```python
from build123d import *

# Parameters (mm, degrees)
SKETCH2_R           = 1.5
BOSS_EXTRUDE1_DEPTH = 23.04
FILLET1_R           = 0.1


with BuildPart() as part:
    # Sketch1 → Revolve1 (revolve)
    with BuildSketch(Plane(origin=(0, 0, 0), x_dir=(0, 0, -1), z_dir=(1, 0, 0))):
        Polygon((618.283966683, 10.92855784), (618.283966683, 7.778306403), (647.128456403, 7.778306403), (647.128456403, 60.052791184), (640.335726742, 60.052791184), (640.335726742, 55.130523314), (637.579256734, 55.130523314), align=None)
    revolve(axis=Axis((0, 60.052791184, -647.128456403), (0, -1, 0)))

    # Sketch2 → Boss-Extrude1 (add)
    with BuildSketch(Plane(origin=(0, 60.052791184, 0), x_dir=(1, 0, 0), z_dir=(0, 1, 0))):
        with Locations(Location((0, 651.328456403, 0), (0, 0, 90))):
            Circle(SKETCH2_R)
        with Locations(Location((-4.2, 647.128456403, 0), (0, 0, 90))):
            Circle(SKETCH2_R)
        with Locations(Location((0, 642.928456403, 0), (0, 0, 90))):
            Circle(SKETCH2_R)
        with Locations(Location((4.2, 647.128456403, 0), (0, 0, 90))):
            Circle(SKETCH2_R)
    extrude(amount=BOSS_EXTRUDE1_DEPTH)

    # Fillet1
    fillet1_edges = [part.edges().sort_by_distance(p)[0] for p in [
        (0, 60.052791184, -641.428456403),
    ]]
    fillet(fillet1_edges, radius=FILLET1_R)


solid = part.part
```
Work out the finished part from the listing and answer in its coordinate system (mm). A direction names the side the tool comes from. Round coordinates to 2 decimals unless told otherwise and drop trailing zeros. Write each loop counter-clockwise with the first axis right and the second up, starting at its lowest first coordinate (ties: lowest second). Pieces come first, ordered by that corner, then holes.
1) Which of the six approach directions +Z, -Z, +X, -X, +Y, -Y give full straight-line access (tool end or side, diameter ignored) to faces 4 (the face through (-4.65, 71.41, -648.56)), 5 (the face through (0, 7.778, -648))?
2) Consider probe 1 along Y at (x, z) = (-22, -639); probe 2 along Y at (x, z) = (-20.5, -656); probe 3 along X at (y, z) = (23, -629). Determine where each line is inside the solid, lowest interval first.
3) Flat-ended cylindrical pins translate along their axes: P1, Ø8, axis at x = -8, z = -642, coming from the +Y side; P2, Ø10, axis at x = -8, y = 22.5, coming from the +Z side; P3, Ø3, axis at x = -7.5, y = 37, coming from the +Z side. Find the tip coordinate at first contact, or state that the pin passes through.
4) A cutting plane is placed at C-C on y = 48.5. Determine the outline of the cut face in (x, z), and give its area (3 significant figures).
5) A cutting plane is placed at A-A on x = 0. Determine the outline of the cut face in (y, z).
6) Determine the mould class of faces 1 (the face through (0, 83.093, -651)), 2 (the face through (-0.07, 71.46, -641.43)), 3 (the face through (0, 60.053, -647)) for opening direction X: pulls with the +X half, pulls with the -X half, needs draft (parallel to the pull), parting line crosses it, or undercut.
7) A cutting plane is placed at B-B on y = 65.5. Determine the outline of the cut face in (x, z), and give its area (3 significant figures).
Entries:
1. face 4: +Y
1. face 5: +Z, -Z, +X, -X, -Y
2. probe 1: y = 7.78 to 23.28
2. probe 2: y = 7.78 to 25.84
2. probe 3: x = -15.07 to 15.07
3. P1: stops at y = 60.05
3. P2: stops at z = -622.04
3. P3: stops at z = -630.39
4. outline: circle Ø24.89 at (0, -647.13)
4. area: 486 mm2
5. outline: (7.78, -675.97) - (10.93, -675.97) - (55.13, -656.68) - (55.13, -653.92) - (60.05, -653.92) - (60.05, -652.83) - (83.09, -652.83) - (83.09, -649.83) - (60.05, -649.83) - (60.05, -644.53) arc R0.1 cw to (60.15, -644.43) - (83.09, -644.43) - (83.09, -641.43) - (60.15, -641.43) arc R0.1 cw to (60.05, -641.33) - (60.05, -640.34) - (55.13, -640.34) - (55.13, -637.58) - (10.93, -618.28) - (7.78, -618.28) - close
6. face 1: needs draft
6. face 2: parting line crosses it
6. face 3: undercut
7. outline: circle Ø3 at (-4.2, -647.13); circle Ø3 at (0, -651.33); circle Ø3 at (0, -642.93); circle Ø3 at (4.2, -647.13)
7. area: 28.3 mm2
